Can you work these out from the model? Positions are in its coordinate system, mm. Face numbers are marked on the shaded views. Coordinates: 2 decimals unless noted, no trailing zeros. Order: outer loops, then holes, each group sorted by start corner. A loop starts at its lowest first (then second) coordinate and runs counter-clockwise, first axis right, second up. Notation, with made-up numbers: (-40, 30.25) -> (15, 30.25) arc R23 ccw to (15, 65.25) -> close; hole circle Ø3 at (-24.75, 79.5). An arc over 180 degrees is marked (long way). Use a Markdown table: item, result. Add a question column.
1. If I drill on line 1 along Z through (x, y) = (0, 5.5); line 2 along X through (y, z) = (18.25, 9); line 3 along X through (y, z) = (18.25, -7.5), over which ranges is the centre line in solid material (lowest first)? Write a range as from..to.
2. We'd pull the mould along X, two halves only. Please class the marked faces 1, 2 and 3: pulls with the +X half, pulls with the -X half, needs draft (parallel to the pull), parting line crosses it, or undercut.
3. Suppose I cut it at C-C, the plane y = 10.5. List the corners of the cut face in (x, z) for me.
4. Suppose I cut it at B-B, the plane z = 0. List the corners of the cut face in (x, y) for me.
5. Suppose I cut it at A-A, the plane x = 0. List the corners of the cut face in (y, z) for me, then the cut area to 3 significant figures.
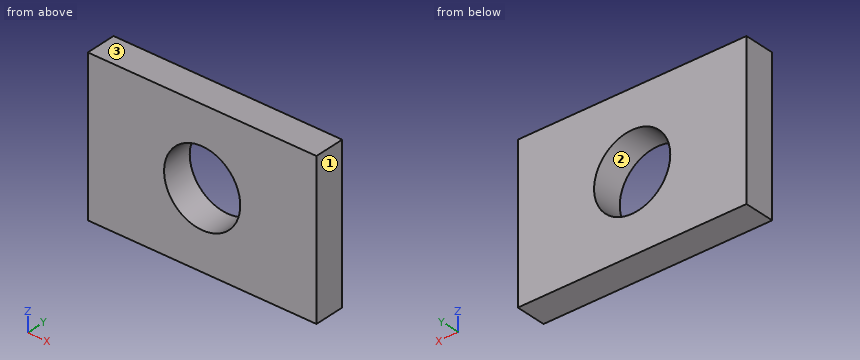
Autodesk Fusion 360 part; units mm, degrees
sketch "Sketch1" plane through (0, 0, 0) normal (0, 1, 0) x (1, 0, 0)
  line L0 (75, 50) -> (-75, 50)
  line L1 (-75, 50) -> (-75, -50)
  line L2 (-75, -50) -> (75, -50)
  line L3 (75, -50) -> (75, 50)
  line L4 (75, 50) -> (-75, -50) construction
  line L5 (-75, 50) -> (75, -50) construction
extrude "Extrude1" add sketch "Sketch1" along normal blind 20
sketch "Sketch2" plane through (0, 20, 0) normal (0, 1, 0) x (-1, 0, 0)
  line L0 (-75, 50) -> (-75, -50)
  line L1 (-75, -50) -> (75, -50)
  line L2 (75, -50) -> (75, 50)
  line L3 (75, 50) -> (-75, 50)
  circle A0 centre (0, 0) radius 25
extrude "Extrude2" cut sketch "Sketch2" against normal blind 20 contours A0
Worked out:
| question | item | result |
|---|---|---|
| 1 | line 1 | z = -50..-25, 25..50 |
| 1 | line 2 | x = -75..-23.32, 23.32..75 |
| 1 | line 3 | x = -75..-23.85, 23.85..75 |
| 2 | face 1 | pulls with the +X half |
| 2 | face 2 | undercut |
| 2 | face 3 | needs draft |
| 3 | outline | (-75, -50) -> (75, -50) -> (75, 50) -> (-75, 50) -> close; hole circle Ø50 at (0, 0) |
| 4 | outline | (-75, 0) -> (-25, 0) -> (-25, 20) -> (-75, 20) -> close; (25, 0) -> (75, 0) -> (75, 20) -> (25, 20) -> close |
| 5 | outline | (0, -50) -> (20, -50) -> (20, -25) -> (0, -25) -> close; (0, 25) -> (20, 25) -> (20, 50) -> (0, 50) -> close |
| 5 | area | 1,000 mm² |
